Geometry: final body of the model. Coordinates: model frame, mm. Round coordinates to 2 decimals unless told otherwise and drop trailing zeros. Order: outer loops, then holes, each group sorted by start corner. A loop starts at its lowest first (then second) coordinate and runs counter-clockwise, first axis right, second up. Notation, with made-up numbers: M 0,65 L 14,65 A30 ccw 14,92 Z; hole C -6,27 d3. An arc over 180 degrees is marked long. Put each result on its own line as item: value. Start each with the question number.
1) First-contact query: P1, Ø3.5, axis at x = -101, z = 0, coming from the -Y side (3 decimals). Flat tip, straight axial feed; report the tip coordinate or a pass-through.
2) Material intervals for probe 1 along Z at (x, y) = (-90, 1.1); probe 2 along X at (y, z) = (0.95, 0); probe 3 along Z at (x, y) = (-101, 1.6), sorted ascending. Write a range as [from, to].
3) Section A-A, the plane x = -90. Return loops of the section in (y, z), then the cut area to 3 significant figures.
4) Section B-B, the plane z = 11. Return loops of the section in (x, y), then the cut area to 3 significant figures.
5) Section C-C, the plane y = 0.7. Return loops of the section in (x, z), then the cut area to 3 significant figures.
6) Section D-D, the plane z = 0. Return loops of the section in (x, y), then the cut area to 3 significant figures.
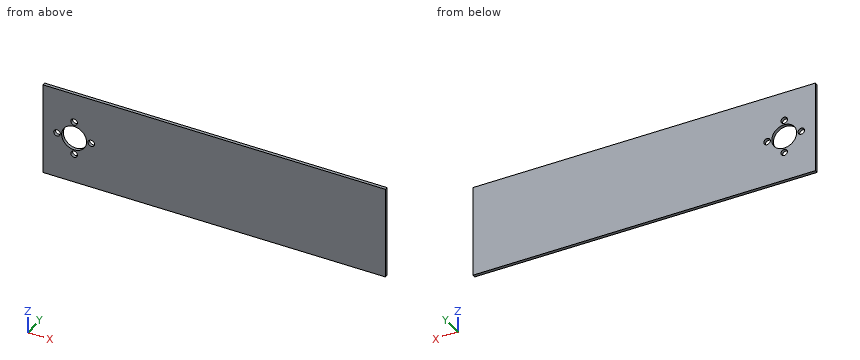
Autodesk Inventor part; units mm, degrees
ref_plane "YZ Plane" through (0, 0, 0) normal (1, 0, 0) x (0, 1, 0)
ref_plane "XZ Plane" through (0, 0, 0) normal (0, 1, 0) x (-1, 0, 0)
ref_plane "XY Plane" through (0, 0, 0) normal (0, 0, 1) x (1, 0, 0)
sketch "スケッチ1" plane through (0, 0, 0) normal (0, 1, 0) x (-1, 0, 0)
  line L0 (-110, -30) -> (110, -30)
  line L1 (110, -30) -> (110, 30)
  line L2 (110, 30) -> (-110, 30)
  line L3 (-110, 30) -> (-110, -30)
  line L4 (-110, -30) -> (110, 30) construction
  line L5 (110, -30) -> (-110, 30) construction
  point P0 (0, 0)
  dimension "d0" = 220
  dimension "d1" = 60
extrude "押し出し1" add sketch "スケッチ1" along normal blind 2
sketch "スケッチ2" plane through (0, 2, 0) normal (0, 1, 0) x (1, 0, 0)
  circle A0 centre (-90, 0) radius 8
  circle A1 centre (-101, 0) radius 2.1
  circle A2 centre (-90, 11) radius 2.1
  circle A3 centre (-79, 0) radius 2.1
  circle A4 centre (-90, -11) radius 2.1
  point P0 (0, 0)
  dimension "d4" = 16
  dimension "d5" = 90
  dimension "d7" = 4.2
  dimension "d8" = 4.2
  dimension "d9" = 4.2
  dimension "d10" = 4.2
  dimension "d13" = 11
  dimension "d14" = 11
  dimension "d15" = 11
  dimension "d16" = 11
extrude "押し出し2" cut sketch "スケッチ2" against normal blind 8
properties part number "snap" material "アルミニウム 6061"
Result sheet:
1. P1: passes through
2. probe 1: z = [-30, -13.1], [-8.9, -8], [8, 8.9], [13.1, 30]
2. probe 2: x = [-110, -103.1], [-98.9, -98], [-82, -81.1], [-76.9, 110]
2. probe 3: z = [-30, -2.1], [2.1, 30]
3. outline: M 0,-30 L 2,-30 L 2,-13.1 L 0,-13.1 Z; M 0,-8.9 L 2,-8.9 L 2,-8 L 0,-8 Z; M 0,8 L 2,8 L 2,8.9 L 0,8.9 Z; M 0,13.1 L 2,13.1 L 2,30 L 0,30 Z
3. area: 71.2 mm2
4. outline: M -110,0 L -92.1,0 L -92.1,2 L -110,2 Z; M -87.9,0 L 110,0 L 110,2 L -87.9,2 Z
4. area: 432 mm2
5. outline: M -110,-30 L 110,-30 L 110,30 L -110,30 Z; hole C -101,0 d4.2; hole C -90,0 d16; hole C -90,-11 d4.2; hole C -90,11 d4.2; hole C -79,0 d4.2
5. area: 12,900 mm2
6. outline: M -110,0 L -103.1,0 L -103.1,2 L -110,2 Z; M -98.9,0 L -98,0 L -98,2 L -98.9,2 Z; M -82,0 L -81.1,0 L -81.1,2 L -82,2 Z; M -76.9,0 L 110,0 L 110,2 L -76.9,2 Z
6. area: 391 mm2
